Geometry check sheet. Reference: the model listing, model coordinates, mm. A direction names the side the tool comes from. Give positions to 0.01 mm unless a question says otherwise; leave off trailing zeros. Loops run counter-clockwise (first coordinate to the right, second up) from the corner with the lowest first, then second, coordinate; pieces in that order, holes last. Notation, with made-up numbers: (89, -37.75) -> (137, -37.75) arc R22 ccw to (137, -31.75) -> close; hole circle Ø5 at (-4.5, -8). An arc over 180 degrees is marked (long way). One line per item, written item: value. Start each with the question number.
(1) Sectioned sample at A-A, the plane x = -19. Record the cut outline in (y, z).
(2) Sectioned sample at C-C, the plane z = -25. Record the cut outline in (x, y).
(3) Sectioned sample at D-D, the plane x = -11. Record the cut outline in (y, z).
(4) Sectioned sample at B-B, the plane y = 42.5. Record the cut outline in (x, z), then the cut area to 3 significant figures.
(5) Draft check along Z on faces 5 (the face through (-20.5, -27, 0)), 6 (the face through (21.5, -37.5, -0.2)), 7 (the face through (16, 43, 25)). Enter one of: pulls with the +Z half, pulls with the -Z half, needs draft (parallel to the pull), parting line crosses it, or undercut.
(6) Gauge pin test, flat ends, axial feed: pin 1 Ø1.5 at (x, z) = (-10, 12) entering from -Y; pin 2 Ø7 at (x, y) = (18, 5) entering from +Z; pin 3 Ø3.5 at (y, z) = (50.5, 25) entering from +X. Record the tip position at first contact, or that the pin passes through.
(7) Tool access check on faces 1 (the face through (16, 28, -16)), 2 (the face through (-17.542, -33.494, 0.264)), 3 (the face through (-20, 29.5, 0)), 4 (the face through (-21, 43, 11)). Record the directions out of +Z, -Z, +X, -X, +Y, -Y that give a thin tool (end or side, any length) a straight path to the whole face; none if there is none.
(8) Scan lines: line 1 along Z through (x, y) = (-17, 34.5); line 2 along Y through (x, z) = (3, -22); line 3 along Z through (x, y) = (-17.2, -27.5). Record each from-to range of solid material in increasing order. Write a range as from..to.
from build123d import *

# Parameters (mm, degrees)
F1_DEPTH  = 10
F2_R      = 10
F3_DEPTH  = 2
F5_DEPTH  = 2
F6_R      = 6
F6_R_2    = 4
F7_DEPTH  = 6
F8_R      = 6
F9_DEPTH  = 3
F10_W     = 32
F10_H     = 17.5
F11_DEPTH = 2
F13_DEPTH = 6
F15_DEPTH = 6
F16_R     = 1.5
F17_DEPTH = 50.8
F18_R     = 1.5
F19_DEPTH = 50.8
F20_W     = 2
F20_H     = 30
F21_DEPTH = 43
F22_R     = 4
F23_DEPTH = 3


with BuildPart() as f1:
    # F0 (on Top) → F1 (new body, symmetric)
    with BuildSketch(Plane.XY):
        Polygon((22.5, -27.5), (22.5, 29.5), (-22.5, 29.5), (-22.5, -27.5), (-20.5, -27.5), (-20.5, 27.5), (20.5, 27.5), (20.5, -27.5), align=None)
    extrude(amount=F1_DEPTH, both=True)

    # F2 (on face) → F3 (join)
    with BuildSketch(Plane(origin=(-22.5, 0, 0), x_dir=(0, -1, 0), z_dir=(-1, 0, 0))):
        with Locations((27.5, 0)):
            Circle(F2_R)
    extrude(amount=-F3_DEPTH)

    # F4 (on face) → F5 (join)
    with BuildSketch(Plane(origin=(20.5, 0, 0), x_dir=(0, -1, 0), z_dir=(-1, 0, 0))):
        with BuildLine():
            Line((27.5, 10), (27.5, -10))
            ThreePointArc((27.5, -10), (37.5, 0), (27.5, 10))
        make_face()
    extrude(amount=-F5_DEPTH)

    # F6 (on face) → F7 (join)
    with BuildSketch(Plane.YZ.offset(-20.5)):
        with Locations((-27.5, 0)):
            Circle(F6_R)
        with Locations((-27.5, 0)):
            Circle(F6_R_2, mode=Mode.SUBTRACT)
    extrude(amount=F7_DEPTH)

    # F8 (on face) → F9 (join)
    with BuildSketch(Plane(origin=(20.5, 0, 0), x_dir=(0, -1, 0), z_dir=(-1, 0, 0))):
        with Locations((27.5, 0)):
            Circle(F8_R)
    extrude(amount=F9_DEPTH)

    # F10 (on face) → F11 (join)
    with BuildSketch(Plane.XZ.offset(-27.5)):
        with Locations((0, -18.75)):
            Rectangle(F10_W, F10_H)
        with Locations((0, 18.75)):
            Rectangle(F10_W, F10_H)
    extrude(amount=-F11_DEPTH)

    # F12 (on face) → F13 (join)
    with BuildSketch(Plane(origin=(0, 0, -27.5), x_dir=(1, 0, 0), z_dir=(0, 0, -1))):
        Polygon((18, -57.5), (18, -27.5), (16, -27.5), (16, -29.5), (16, -55.5), (-16, -55.5), (-16, -29.5), (-16, -27.5), (-18, -27.5), (-18, -57.5), align=None)
    extrude(amount=-F13_DEPTH)

    # F14 (on face) → F15 (join)
    with BuildSketch(Plane.XY.offset(27.5)):
        Polygon((-16, 27.5), (-16, 55.5), (16, 55.5), (16, 27.5), (18, 27.5), (18, 57.5), (-18, 57.5), (-18, 27.5), align=None)
    extrude(amount=-F15_DEPTH)

    # F16 (on face) → F17 (cut)
    with BuildSketch(Plane(origin=(-18, 0, 0), x_dir=(0, -1, 0), z_dir=(-1, 0, 0))):
        with Locations((-50.5, 25)):
            Circle(F16_R)
        with Locations((-34.5, 25)):
            Circle(F16_R)
    extrude(amount=-F17_DEPTH, mode=Mode.SUBTRACT)

    # F18 (on face) → F19 (cut)
    with BuildSketch(Plane(origin=(-18, 0, 0), x_dir=(0, -1, 0), z_dir=(-1, 0, 0))):
        with Locations((-50.5, -25)):
            Circle(F18_R)
        with Locations((-34.5, -25)):
            Circle(F18_R)
    extrude(amount=-F19_DEPTH, mode=Mode.SUBTRACT)

    # F20 (on face) → F21 (join)
    with BuildSketch(Plane(origin=(0, 0, 21.5), x_dir=(1, 0, 0), z_dir=(0, 0, -1))):
        with Locations((-17, -42.5)):
            Rectangle(F20_W, F20_H)
    extrude(amount=F21_DEPTH)

    # F22 (on face) → F23 (join)
    with BuildSketch(Plane(origin=(-18, 0, 0), x_dir=(0, -1, 0), z_dir=(-1, 0, 0))):
        with Locations((-42.5, 11)):
            Circle(F22_R)
        with Locations((-42.5, -11)):
            Circle(F22_R)
    extrude(amount=F23_DEPTH)


solid = f1.part
Calculated:
1. outline: circle Ø12 at (-27.5, 0); (27.5, -10) -> (29.5, -10) -> (29.5, 10) -> (27.5, 10) -> close; circle Ø8 at (42.5, -11); circle Ø8 at (42.5, 11); hole circle Ø8 at (-27.5, 0)
2. outline: (-18, 27.5) -> (18, 27.5) -> (18, 33) -> (16, 33) -> (16, 29.5) -> (-16, 29.5) -> (-16, 33) -> (-18, 33) -> close; (-18, 36) -> (-16, 36) -> (-16, 49) -> (-18, 49) -> close; (-18, 52) -> (-16, 52) -> (-16, 55.5) -> (16, 55.5) -> (16, 52) -> (18, 52) -> (18, 57.5) -> (-18, 57.5) -> close; (16, 36) -> (18, 36) -> (18, 49) -> (16, 49) -> close
3. outline: (27.5, -27.5) -> (29.5, -27.5) -> (29.5, 27.5) -> (27.5, 27.5) -> close; (55.5, -27.5) -> (57.5, -27.5) -> (57.5, -21.5) -> (55.5, -21.5) -> close; (55.5, 21.5) -> (57.5, 21.5) -> (57.5, 27.5) -> (55.5, 27.5) -> close
4. outline: (-21, -15) -> (-18, -15) -> (-18, -27.5) -> (-16, -27.5) -> (-16, 27.5) -> (-18, 27.5) -> (-18, 15) -> (-21, 15) -> (-21, 7) -> (-18, 7) -> (-18, -7) -> (-21, -7) -> close; (16, -27.5) -> (18, -27.5) -> (18, -21.5) -> (16, -21.5) -> close; (16, 21.5) -> (18, 21.5) -> (18, 27.5) -> (16, 27.5) -> close
4. area: 182 mm2
5. face 5: undercut
5. face 6: parting line crosses it
5. face 7: needs draft
6. pin 1: stops at y = 27.5
6. pin 2: stops at z = 10
6. pin 3: stops at x = 18
7. face 1: +X, +Y, -Y
7. face 2: none
7. face 3: +Z, -Z, -X
7. face 4: +Z, -Z, -X, +Y
8. line 1: z = -27.5..-26.5, -23.5..23.5, 26.5..27.5
8. line 2: y = 27.5..29.5, 55.5..57.5
8. line 3: z = -6..-4, 4..6
